CAD build for the part. Positions are in the model's coordinates, mm. Give positions to 0.01 mm unless a question says otherwise; leave off trailing zeros. Order: outer loops, then holes, each group sorted by start corner. A loop starts at its lowest first (then second) coordinate and runs counter-clockwise, first axis right, second up.
Item 1: Wall check: L1, parallel to X at y = 4, z = 10; L2, parallel to X at y = 0, z = 1.75; L3, parallel to Y at x = -3, z = 12. Give the ranges that are in metal, low to high.
Item 2: Band-saw the part on B-B on x = -5. Give the cut face in (y, z), plus the area to 3 significant figures.
Item 3: Two-plate mould, pull along Y, no slides. Class faces 1 (the cylindrical face through (-4.23, -2.95, 9.39)), 2 (the flat face through (-13.962, 23, 10)), 3 (the cylindrical face through (-1.44, 1.69, 9.39)): released by +Y, released by -Y, zero draft, split by the parting line, or undercut.
Item 4: Band-saw the part on C-C on z = 11. Give the cut face in (x, y) (3 decimals), plus the area to 3 significant figures.
Item 5: Band-saw the part on D-D on x = 3.25. Give the cut face in (y, z).
Item 6: Flat gauge pin, fed straight in: P1, Ø6, axis at x = -12, z = 14, coming from the -Y side. Where does the tip first touch, or does it go through?
Item 7: Band-saw the part on A-A on y = 3. Give the cut face in (x, z), plus the area to 3 significant figures.
```python
from build123d import *

# Parameters (mm, degrees)
SKETCH1_R           = 3
BOSS_EXTRUDE1_DEPTH = 19.05
SKETCH3_W           = 19.05
SKETCH3_H           = 19.05
BOSS_EXTRUDE2_DEPTH = 25.4


with BuildPart() as part:
    # Sketch1 → Boss-Extrude1 (new body)
    with BuildSketch(Plane.XY):
        with BuildLine():
            Line((-13.962302658, 14.995513055), (5.087697342, 14.995513055))
            Line((5.087697342, 14.995513055), (5.087697342, 6.570840919))
            ThreePointArc((5.087697342, 6.570840919), (-4.437302658, -2.954159081), (-13.962302658, 6.570840919))
            Line((-13.962302658, 6.570840919), (-13.962302658, 14.995513055))
        make_face()
        with Locations(Location((-4.437302658, 1.820065848, 0), (0, 0, 180))):
            Circle(SKETCH1_R, mode=Mode.SUBTRACT)
    extrude(amount=BOSS_EXTRUDE1_DEPTH)

    # Sketch3 → Boss-Extrude2 (add)
    with BuildSketch(Plane(origin=(0, 14.995513055, 0), x_dir=(1, 0, 0), z_dir=(0, 1, 0))):
        with Locations((-4.437302658, -9.525)):
            Rectangle(SKETCH3_W, SKETCH3_H)
    extrude(amount=BOSS_EXTRUDE2_DEPTH)


solid = part.part
```
The answers:
1. L1: x = -13.61 to -6.5, -2.38 to 4.73
1. L2: x = -11.33 to -6.82, -2.05 to 2.46
1. L3: y = -2.85 to -0.81, 4.45 to 40.4
2. outline: (-2.94, 0) - (-1.13, 0) - (-1.13, 19.05) - (-2.94, 19.05) - close; (4.77, 0) - (40.4, 0) - (40.4, 19.05) - (4.77, 19.05) - close
2. area: 713 mm2
3. face 1: released by -Y
3. face 2: zero draft
3. face 3: undercut
4. outline: (-13.962, 6.571) arc R9.525 ccw to (5.088, 6.571) - (5.088, 40.396) - (-13.962, 40.396) - close; hole circle Ø6 at (-4.437, 1.82)
4. area: 759 mm2
5. outline: (0.95, 0) - (40.4, 0) - (40.4, 19.05) - (0.95, 19.05) - close
6. P1: stops at y = -1.79
7. outline: (-13.27, 0) - (-7.2, 0) - (-7.2, 19.05) - (-13.27, 19.05) - close; (-1.68, 0) - (4.39, 0) - (4.39, 19.05) - (-1.68, 19.05) - close
7. area: 231 mm2
